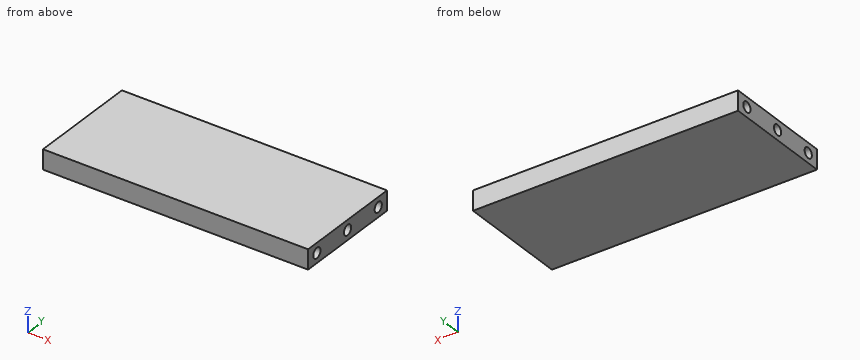
```python
from build123d import *

# Parameters (mm, degrees)
SKETCH1_W           = 86
SKETCH1_H           = 36
BOSS_EXTRUDE1_DEPTH = 3.175
SKETCH2_R           = 1.65
CUT_EXTRUDE1_DEPTH  = 10


with BuildPart() as part:
    # Sketch1 → Boss-Extrude1 (new, symmetric)
    with BuildSketch(Plane.XY):
        Rectangle(SKETCH1_W, SKETCH1_H)
    extrude(amount=BOSS_EXTRUDE1_DEPTH, both=True)

    # Sketch2 → Cut-Extrude1 (cut)
    with BuildSketch(Plane.ZY.offset(43)):
        with Locations((0, 14)):
            Circle(SKETCH2_R)
        with Locations((0, -14)):
            Circle(SKETCH2_R)
        Circle(SKETCH2_R)
    cut_extrude1 = extrude(amount=-CUT_EXTRUDE1_DEPTH, mode=Mode.SUBTRACT)

    # Mirror1: Cut-Extrude1 across plane
    add(cut_extrude1.mirror(Plane(origin=(0, 0, 0), x_dir=(0, 0, 1), z_dir=(1, 0, 0))), mode=Mode.SUBTRACT)


solid = part.part
```
Here's how the part is built. I have some questions about the finished solid (model axes, mm). Round coordinates to 2 decimals unless told otherwise and drop trailing zeros. Order: outer loops, then holes, each group sorted by start corner. A loop starts at its lowest first (then second) coordinate and runs counter-clockwise, first axis right, second up. Notation, with made-up numbers: M -13,68.25 L 8,68.25 A16 ccw 8,99.25 Z; hole C 83,-5 d8. An arc over 180 degrees is marked long. Answer in a Markdown table with one row per item.
Item 1: I'm going to push flat-ended pins straight in: pin 1 (1.6 mm diameter, centred on y = 14.5, z = 0, fed in from +X); pin 2 (1 mm diameter, centred on y = -13.5, z = 0, fed in from -X). Where does each tip first touch, or does it pass through?
A:
| item | result |
|---|---|
| pin 1 | stops at x = 33 |
| pin 2 | stops at x = -33 |
Item 2: If I drill on L1, parallel to Y at x = 38.75, z = 0; L2, parallel to X at y = -1, z = 0.5, over which ranges is the centre line in solid material (lowest first)? Write a range as from..to.
A:
| item | result |
|---|---|
| L1 | y = -18..-15.65, -12.35..-1.65, 1.65..12.35, 15.65..18 |
| L2 | x = -33..33 |
Item 3: Imagine slicing it at A-A, the plane y = -14. Write out the boundary of the cut face in (x, z) (3 decimals), and give its area (3 significant figures).
A:
| item | result |
|---|---|
| outline | M -43,-3.175 L 43,-3.175 L 43,-1.65 L 33,-1.65 L 33,1.65 L 43,1.65 L 43,3.175 L -43,3.175 L -43,1.65 L -33,1.65 L -33,-1.65 L -43,-1.65 Z |
| area | 480 mm2 |
Item 4: Imagine slicing it at B-B, the plane z = 0. Write out the boundary of the cut face in (x, y).
A:
| item | result |
|---|---|
| outline | M -43,-18 L 43,-18 L 43,-15.65 L 33,-15.65 L 33,-12.35 L 43,-12.35 L 43,-1.65 L 33,-1.65 L 33,1.65 L 43,1.65 L 43,12.35 L 33,12.35 L 33,15.65 L 43,15.65 L 43,18 L -43,18 L -43,15.65 L -33,15.65 L -33,12.35 L -43,12.35 L -43,1.65 L -33,1.65 L -33,-1.65 L -43,-1.65 L -43,-12.35 L -33,-12.35 L -33,-15.65 L -43,-15.65 Z |
